from build123d import *

# Parameters (mm, degrees)
F1_DEPTH = 4


with BuildPart() as f1:
    # F0 (on Top) → F1 (new body)
    with BuildSketch(Plane.XY):
        with BuildLine():
            Line((0, 100), (-42.1617882956, 50))
            ThreePointArc((-42.1617882956, 50), (-37.1768676119, 47.106612997), (-31.994432446, 44.5840174441))
            ThreePointArc((-31.994432446, 44.5840174441), (-21.0663934766, 40.6801499068), (-9.6846764242, 38.4176878845))
            ThreePointArc((-9.6846764242, 38.4176878845), (0.15722732, 37.8225468215), (9.9966866024, 38.4568205982))
            ThreePointArc((9.9966866024, 38.4568205982), (21.2178970455, 40.7221870715), (31.994432446, 44.5840174441))
            ThreePointArc((31.994432446, 44.5840174441), (37.1768676119, 47.106612997), (42.1617882956, 50))
            Line((42.1617882956, 50), (0, 100))
        make_face()
        with BuildLine():
            ThreePointArc((-9.6846764242, 38.4176878845), (-21.0663934766, 40.6801499068), (-31.994432446, 44.5840174441))
            Line((-31.994432446, 44.5840174441), (-64.382164337, 0))
            ThreePointArc((-64.382164337, 0), (-57.0326259859, -3.8851908994), (-49.4497308534, -7.2925540604))
            Line((-49.4497308534, -7.2925540604), (-9.6846764242, 38.4176878845))
        make_face()
        with BuildLine():
            ThreePointArc((9.9966866024, 38.4568205982), (0.15722732, 37.8225468215), (-9.6846764242, 38.4176878845))
            Line((-9.6846764242, 38.4176878845), (-49.4497308534, -7.2925540604))
            ThreePointArc((-49.4497308534, -7.2925540604), (0.0665901335, -17.0676588152), (49.5728681141, -7.2418175004))
            Line((49.5728681141, -7.2418175004), (9.9966866024, 38.4568205982))
        make_face()
        with BuildLine():
            ThreePointArc((31.994432446, 44.5840174441), (21.2178970455, 40.7221870715), (9.9966866024, 38.4568205982))
            Line((9.9966866024, 38.4568205982), (49.5728681141, -7.2418175004))
            ThreePointArc((49.5728681141, -7.2418175004), (57.0924542774, -3.8559535654), (64.382164337, 0))
            Line((64.382164337, 0), (31.994432446, 44.5840174441))
        make_face()
        with BuildLine():
            ThreePointArc((49.5728681141, -7.2418175004), (0.0665901335, -17.0676588152), (-49.4497308534, -7.2925540604))
            Line((-49.4497308534, -7.2925540604), (-86.6025403784, -50))
            ThreePointArc((-86.6025403784, -50), (-56.9443850461, -69.4774247767), (-23.1684497457, -80.347679982))
            Line((-23.1684497457, -80.347679982), (-23.1684497457, -50))
            Line((-23.1684497457, -50), (23.1684497457, -50))
            Line((23.1684497457, -50), (23.1684497457, -80.347679982))
            ThreePointArc((23.1684497457, -80.347679982), (56.9443850461, -69.4774247767), (86.6025403784, -50))
            Line((86.6025403784, -50), (49.5728681141, -7.2418175004))
        make_face()
        with BuildLine():
            Line((-23.1684497457, -50), (-23.1684497457, -80.347679982))
            ThreePointArc((-23.1684497457, -80.347679982), (0, -82.3976528812), (23.1684497457, -80.347679982))
            Line((23.1684497457, -80.347679982), (23.1684497457, -50))
            Line((23.1684497457, -50), (-23.1684497457, -50))
        make_face()
        with BuildLine():
            ThreePointArc((23.1684497457, -80.347679982), (0, -82.3976528812), (-23.1684497457, -80.347679982))
            Line((-23.1684497457, -80.347679982), (-23.1684497457, -96.3368994915))
            Line((-23.1684497457, -96.3368994915), (23.1684497457, -96.3368994915))
            Line((23.1684497457, -96.3368994915), (23.1684497457, -80.347679982))
        make_face()
    extrude(amount=F1_DEPTH)


solid = f1.part
Source: CAD feature listing. Evaluate the final solid. Frame: model axes, mm. A direction names the side the tool comes from. Coordinates: 2 decimals unless noted, no trailing zeros. Loops run counter-clockwise (first coordinate to the right, second up) from the corner with the lowest first, then second, coordinate; pieces in that order, holes last. Notation, with made-up numbers: M 80,-23.5 L 123,-23.5 A27 cw 123,2.5 Z; hole C 51,-8.5 d9. An arc over 180 degrees is marked long. Answer in a Markdown table with one row per item.
Q1. Section D-D on x = -27.5. Return the cut outline in (y, z), plus the area to 3 significant figures.
Answers below:
| item | result |
|---|---|
| outline | M -79.5,0 L 67.39,0 L 67.39,4 L -79.5,4 Z |
| area | 588 mm^2 |
Q2. First-contact query: pin 1 (2 mm diameter, centred on y = -91.5, z = 1, fed in from -X). Flat tip, straight axial feed; report the tip coordinate or a pass-through.
Answers below:
| item | result |
|---|---|
| pin 1 | stops at x = -23.17 |
Q3. Draft query along Y for faces 6 (the flat face through (-20.786, 75.35, 1.972)), 7 (the flat face through (-1, -19, 0)), 8 (the cylindrical face through (37.11, 47.07, 1.97)), 9 (the flat face through (68.347, -28.92, 1.972)). Return one class per face: pulls with the +Y half, pulls with the -Y half, needs draft (parallel to the pull), parting line crosses it, or undercut.
Answers below:
| item | result |
|---|---|
| face 6 | pulls with the +Y half |
| face 7 | needs draft |
| face 8 | undercut |
| face 9 | undercut |
Q4. Set-up query: faces 1 (the flat face through (48.4, 22, 2)), 2 (the flat face through (23.168, -88, 2)), 3 (the flat face through (-23.168, -88, 2)), 4 (the flat face through (-47.962, 22.604, 1.972)), 5 (the flat face through (0, -96.337, 2)). Return all of +Z, -Z, +X, -X, +Y, -Y with unobstructed straight access to the full face (end or side cutting, diameter ignored); none if empty.
Answers below:
| item | result |
|---|---|
| face 1 | +Z, -Z, +X |
| face 2 | +Z, -Z, +X, -Y |
| face 3 | +Z, -Z, -X, -Y |
| face 4 | +Z, -Z, -X |
| face 5 | +Z, -Z, +X, -X, -Y |
Q5. Section A-A on z = 2.2. Return the cut outline in (x, y), plus the area to 3 significant figures.
Answers below:
| item | result |
|---|---|
| outline | M -86.6,-50 A131.95 ccw -23.17,-80.35 L -23.17,-96.34 L 23.17,-96.34 L 23.17,-80.35 A131.95 ccw 86.6,-50 L 49.57,-7.24 A129.96 ccw 64.38,0 L 31.99,44.58 A79.08 ccw 42.16,50 L 0,100 L -42.16,50 A79.08 ccw -31.99,44.58 L -64.38,0 A129.96 ccw -49.45,-7.29 Z |
| area | 18,000 mm^2 |
Q6. Section C-C on y = -64.5. Return the cut outline in (x, z).
Answers below:
| item | result |
|---|---|
| outline | M -66.35,0 L 66.35,0 L 66.35,4 L -66.35,4 Z |
Q7. Section B-B on x = -52. Return the cut outline in (y, z).
Answers below:
| item | result |
|---|---|
| outline | M -71.72,0 L -10.22,0 L -10.22,4 L -71.72,4 Z; M -6.21,0 L 17.04,0 L 17.04,4 L -6.21,4 Z |
Q8. Ray query, probe 1 along Y at (x, z) = (-62.5, 0.6); probe 2 along Y at (x, z) = (-11, 2.45); probe 3 along X at (y, z) = (21, 0.8). Return the intervals inside material, ascending. Write a range as from..to.
Answers below:
| item | result |
|---|---|
| probe 1 | y = -66.66..-22.29, -1.05..2.59 |
| probe 2 | y = -96.34..86.96 |
| probe 3 | x = -49.13..49.13 |
